Work out the finished part from the listing and answer in its coordinate system (mm). A direction names the side the tool comes from. Coordinates: 2 decimals unless noted, no trailing zeros. Order: outer loops, then holes, each group sorted by start corner. A loop starts at its lowest first (then second) coordinate and runs counter-clockwise, first axis right, second up. Notation, with made-up numbers: (6.25, -39) -> (25.25, -39) arc R27 ccw to (25.25, -13) -> close; hole circle Ø10 at (81.25, 69.5). An arc over 180 degrees is marked (long way). Use one line per item in the form item = value.
from build123d import *

# Parameters (mm, degrees)
EXTRUDE1_DEPTH     = 3
SKETCH2_R          = 1.6
CUT_EXTRUDE1_DEPTH = 3


with BuildPart() as part:
    # Sketch1 → Extrude1 (new body)
    with BuildSketch(Plane.XY):
        with BuildLine():
            Line((-512.555561166, 145), (-472.555561166, 145))
            ThreePointArc((-472.555561166, 145), (-455.723951498, 150.166616904), (-444.689840432, 163.886872268))
            Line((-444.689840432, 163.886872268), (-436.785621791, 183.706382542))
            ThreePointArc((-436.785621791, 183.706382542), (-433.10758477, 188.279800996), (-427.497048214, 190.002006631))
            Line((-427.497048214, 190.002006631), (-157.497048214, 190.002006631))
            ThreePointArc((-157.497048214, 190.002006631), (-151.886511658, 188.279800996), (-148.208474636, 183.706382542))
            Line((-148.208474636, 183.706382542), (-140.304255995, 163.886872268))
            ThreePointArc((-140.304255995, 163.886872268), (-129.270144929, 150.166616904), (-112.438535261, 145))
            Line((-112.438535261, 145), (-72.438535261, 145))
            Line((-72.438535261, 145), (-72.438535261, 165))
            Line((-72.438535261, 165), (-112.438535261, 165))
            ThreePointArc((-112.438535261, 165), (-118.049071817, 166.722205635), (-121.727108839, 171.295624089))
            Line((-121.727108839, 171.295624089), (-129.63132748, 191.115134363))
            ThreePointArc((-129.63132748, 191.115134363), (-140.665438546, 204.835389727), (-157.497048214, 210.002006631))
            Line((-157.497048214, 210.002006631), (-427.497048214, 210.002006631))
            ThreePointArc((-427.497048214, 210.002006631), (-444.328657882, 204.835389727), (-455.362768947, 191.115134363))
            Line((-455.362768947, 191.115134363), (-463.266987588, 171.295624089))
            ThreePointArc((-463.266987588, 171.295624089), (-466.94502461, 166.722205635), (-472.555561166, 165))
            Line((-472.555561166, 165), (-512.555561166, 165))
            Line((-512.555561166, 165), (-512.555561166, 145))
        make_face()
    extrude(amount=EXTRUDE1_DEPTH)

    # Sketch2 → Cut-Extrude1 (cut)
    with BuildSketch(Plane.XY.offset(3)):
        with Locations((-494.555561166, 155)):
            Circle(SKETCH2_R)
        with Locations((-464.555561166, 155)):
            Circle(SKETCH2_R)
        with Locations((-427.497048214, 200.002006631)):
            Circle(SKETCH2_R)
        with Locations((-407.497048214, 199.95245399)):
            Circle(SKETCH2_R)
        with Locations((-387.497048214, 199.90290135)):
            Circle(SKETCH2_R)
        with Locations((-504.555561166, 155)):
            Circle(SKETCH2_R)
        with Locations((-80.438535261, 155)):
            Circle(SKETCH2_R)
        with Locations((-197.497048214, 199.90290135)):
            Circle(SKETCH2_R)
        with Locations((-177.497048214, 199.95245399)):
            Circle(SKETCH2_R)
        with Locations((-157.497048214, 200.002006631)):
            Circle(SKETCH2_R)
        with Locations((-120.438535261, 155)):
            Circle(SKETCH2_R)
        with Locations((-90.438535261, 155)):
            Circle(SKETCH2_R)
    extrude(amount=-CUT_EXTRUDE1_DEPTH, mode=Mode.SUBTRACT)


solid = part.part
(1) The mould has two halves that part along X. Classify faces 1 (the flat face through (-125.624, 181.067, 1.479)), 2 (the flat face through (-294, 197, 3)), 3 (the flat face through (-440.793, 173.658, 1.479)): released by +X, released by -X, zero draft, split by the parting line, or undercut.
Data:
face_1 = released by +X
face_2 = zero draft
face_3 = undercut
(2) Each of these flat-tipped pins is pushed along its axis until it touches: P1, Ø1.5, axis at x = -497.5, z = 2, coming from the +Y side; P2, Ø1.9, axis at x = -120.44, y = 155, coming from the -Z side. Where does it stop, or does it pass through?
Data:
P1 = 165
P2 = through
(3) Which of the six approach directions +Z, -Z, +X, -X, +Y, -Y give full straight-line access (tool end or side, diameter ignored) to faces 4 (the cylindrical face through (-444.121, 204.975, 1.479)), 5 (the cylindrical face through (-455.93, 150.03, 1.48))?
Data:
face_4 = +Z, -Z, -X, +Y
face_5 = +Z, -Z, -Y
(4) Straight lines are drawn through the part: line 1 along X through (y, z) = (160.5, 2.7); line 2 along Y through (x, z) = (-200, 2.6); line 3 along X through (y, z) = (184, 1.1). For each, find the intervals that lie inside material, in ascending order.
Data:
line_1 = -512.56 to -446.29, -138.7 to -72.44
line_2 = 190 to 210
line_3 = -458.2 to -436.66, -148.33 to -126.79
(5) Section B-B on x = -356.5 is taken. Write down the section's boundary in (y, z), plus the area to 3 significant figures.
Data:
outline = (190, 0) -> (210, 0) -> (210, 3) -> (190, 3) -> close
area = 60.0 mm²
(6) Section A-A on z = 0.9 is taken. Count the separate pieces of the cut face and the enclosed holes in it, plus the area to 3 significant figures.
Data:
separate_pieces = 1
enclosed_holes = 12
area = 9,660 mm²
